from build123d import *

# Parameters (mm, degrees)
SKETCH1_W                = 89
SKETCH1_H                = 83
SKETCH1_R                = 1.3
MAIN_BODY_DEPTH          = 14
SKETCH2_W                = 40
SKETCH2_H                = 83
SCREW_GROOVE_DEPTH       = 6
SKETCH4_W                = 9
SKETCH4_H                = 83
MOUNT_LIFT_DEPTH         = 20
MOUNT_START              = -5.55625
MOUNT_NUTS_DEPTH         = 18.94375
F_9_32_MOUNT_HOLES_REACH = 7.556
SKETCH5_R                = 3.3734375
SKETCH8_W                = 15.5
SKETCH8_H                = 43
MIDDLE_CUT_DEPTH         = 14


with BuildPart() as part:
    # Sketch1 → Main Body (new body)
    with BuildSketch(Plane(origin=(0, 0, 0), x_dir=(1, 0, 0), z_dir=(0, 1, 0))):
        with Locations((0, 41.5)):
            Rectangle(SKETCH1_W, SKETCH1_H)
        with Locations((-30, 14.25)):
            Circle(SKETCH1_R, mode=Mode.SUBTRACT)
        with Locations((30, 14.25)):
            Circle(SKETCH1_R, mode=Mode.SUBTRACT)
        with BuildLine():
            ThreePointArc((0, 5), (-5.303300859, 7.196699141), (-7.5, 12.5))
            Line((-7.5, 12.5), (-7.5, 63))
            Line((-7.5, 63), (7.5, 63))
            Line((7.5, 63), (7.5, 12.5))
            ThreePointArc((7.5, 12.5), (5.303300859, 7.196699141), (0, 5))
        make_face(mode=Mode.SUBTRACT)
        with Locations((-30, 68.75)):
            Circle(SKETCH1_R, mode=Mode.SUBTRACT)
        with Locations((30, 68.75)):
            Circle(SKETCH1_R, mode=Mode.SUBTRACT)
    extrude(amount=MAIN_BODY_DEPTH)

    # Sketch2 → Screw Groove (cut)
    with BuildSketch(Plane(origin=(0, 14, 0), x_dir=(1, 0, 0), z_dir=(0, 1, 0))):
        with Locations((0, 41.5)):
            Rectangle(SKETCH2_W, SKETCH2_H)
    extrude(amount=-SCREW_GROOVE_DEPTH, mode=Mode.SUBTRACT)

    # Sketch4 → Mount Lift (add)
    with BuildSketch(Plane(origin=(0, 14, 0), x_dir=(1, 0, 0), z_dir=(0, 1, 0))):
        with Locations((-40, 41.5)):
            Rectangle(SKETCH4_W, SKETCH4_H)
        with Locations((40, 41.5)):
            Rectangle(SKETCH4_W, SKETCH4_H)
    extrude(amount=MOUNT_LIFT_DEPTH)

    # Sketch6 → Mount Nuts (cut)
    with BuildSketch(Plane.ZY.offset(44.5).offset(MOUNT_START)):
        Polygon((-52.855059246, 19.7546875), (-56.177529623, 25.509375), (-62.822470377, 25.509375), (-66.144940754, 19.7546875), (-62.822470377, 14), (-56.177529623, 14), align=None)
        Polygon((-16.855059246, 19.7546875), (-20.177529623, 25.509375), (-26.822470377, 25.509375), (-30.144940754, 19.7546875), (-26.822470377, 14), (-20.177529623, 14), align=None)
    extrude(amount=-MOUNT_NUTS_DEPTH, mode=Mode.SUBTRACT)

    # Sketch5 → 9/32 Mount Holes (cut, up to next)
    with BuildSketch(Plane.ZY.offset(38.94375), mode=Mode.PRIVATE) as f_9_32_mount_holes_sk1:
        with Locations((-59.5, 19.7546875)):
            Circle(SKETCH5_R)
    f_9_32_mount_holes_tool1 = extrude(f_9_32_mount_holes_sk1.sketch, amount=F_9_32_MOUNT_HOLES_REACH, mode=Mode.PRIVATE) & part.part
    add(f_9_32_mount_holes_tool1.solids().sort_by_distance((-38.94375, 19.754688, -59.5))[0], mode=Mode.SUBTRACT)
    # Sketch5 → 9/32 Mount Holes (cut, up to next)
    with BuildSketch(Plane.ZY.offset(38.94375), mode=Mode.PRIVATE) as f_9_32_mount_holes_sk2:
        with Locations((-23.5, 19.7546875)):
            Circle(SKETCH5_R)
    f_9_32_mount_holes_tool2 = extrude(f_9_32_mount_holes_sk2.sketch, amount=F_9_32_MOUNT_HOLES_REACH, mode=Mode.PRIVATE) & part.part
    add(f_9_32_mount_holes_tool2.solids().sort_by_distance((-38.94375, 19.754688, -23.5))[0], mode=Mode.SUBTRACT)

    # Sketch8 → Middle Cut (cut)
    with BuildSketch(Plane(origin=(0, 14, 0), x_dir=(1, 0, 0), z_dir=(0, 1, 0))):
        with Locations((-27.75, 41.5)):
            Rectangle(SKETCH8_W, SKETCH8_H)
        with Locations((27.75, 41.5)):
            Rectangle(SKETCH8_W, SKETCH8_H)
    extrude(amount=-MIDDLE_CUT_DEPTH, mode=Mode.SUBTRACT)


solid = part.part
The listing builds one solid part. Answer for the finished solid, in the listing's coordinates (mm). A direction names the side the tool comes from. Round coordinates to 2 decimals unless told otherwise and drop trailing zeros. Write each loop counter-clockwise with the first axis right and the second up, starting at its lowest first coordinate (ties: lowest second). Pieces come first, ordered by that corner, then holes. Notation, with made-up numbers: M -11,0 L 20,0 A15 cw 20,28 Z; hole C 41.25,-6 d4. An arc over 180 degrees is marked long. Write each question's results on one line, items separated by ' | '. Start each with the question number.
Item 1: Which of the six approach directions +Z, -Z, +X, -X, +Y, -Y give full straight-line access (tool end or side, diameter ignored) to faces 3 (the flat face through (-37.25, 16.92, -64.51)), 4 (the flat face through (28, 14, -73)), 5 (the flat face through (35.5, 21, -41)), 6 (the flat face through (-28, 7, -63))?
Item 2: Find section C-C on x = 30. Write down the section's boundary in (y, z).
Item 3: Find section B-B on z = -59.5. Write down the section's boundary in (x, y), and give its area (3 significant figures).
Item 4: Straight lines are drawn through the part: probe 1 along X at (y, z) = (5, -14); probe 2 along Z at (x, y) = (30, 10.25); probe 3 along X at (y, z) = (28, -62.5). For each, find the intervals that lie inside material, in ascending order.
Item 5: Find section A-A on y = 30.5. Write down the section's boundary in (x, z), and give its area (3 significant figures).
Item 6: The mould has two halves that part along X. Classify faces 1 (the flat face through (-37.25, 22.67, -64.46)), 2 (the cylindrical face through (-41.68, 22.6, -21.69)): +X half, -X half, draft (parallel to the pull), parting line (faces both ways), or undercut.
Item 7: Given pin 1 Ø1.6 at (x, z) = (-30, -68.75) entering from -Y; pin 2 Ø4.5 at (x, z) = (-27, -14.5) entering from +Y, each flat-ended and moving along its own axis, determine where each tip first touches the part or whether it passes through.
Item 8: Find section D-D on x = -33. Write down the section's boundary in (y, z).
Answer block:
1) face 3: none | face 4: +Z, -Z, +Y | face 5: +Y | face 6: +Y, -Y
2) outline: M 0,-83 L 14,-83 L 14,-70.05 L 0,-70.05 Z; M 0,-67.45 L 14,-67.45 L 14,-63 L 0,-63 Z; M 0,-20 L 14,-20 L 14,-15.55 L 0,-15.55 Z; M 0,-12.95 L 14,-12.95 L 14,0 L 0,0 Z
3) outline: M -44.5,0 L -35.5,0 L -35.5,14 L -38.94,14 L -38.94,16.38 L -44.5,16.38 Z; M -44.5,23.13 L -38.94,23.13 L -38.94,25.51 L -35.5,25.51 L -35.5,34 L -44.5,34 Z; M -20,0 L -7.5,0 L -7.5,8 L -20,8 Z; M 7.5,0 L 20,0 L 20,8 L 7.5,8 Z; M 35.5,0 L 44.5,0 L 44.5,34 L 35.5,34 Z | area: 735 mm²
4) probe 1: x = -44.5 to -31.28, -28.72 to -7.5, 7.5 to 28.72, 31.28 to 44.5 | probe 2: z = -83 to -70.05, -67.45 to -63, -20 to -15.55, -12.95 to 0 | probe 3: x = -44.5 to -35.5, 35.5 to 44.5
5) outline: M -44.5,-83 L -35.5,-83 L -35.5,0 L -44.5,0 Z; M 35.5,-83 L 44.5,-83 L 44.5,0 L 35.5,0 Z | area: 1,490 mm²
6) face 1: undercut | face 2: draft
7) pin 1: passes through | pin 2: stops at y = 14
8) outline: M 0,-83 L 14,-83 L 14,-63 L 0,-63 Z; M 0,-20 L 14,-20 L 14,0 L 0,0 Z
